from build123d import *

# Parameters (mm, degrees)
SKETCH1_W               = 35
SKETCH1_H               = 54
BOSS_EXTRUDE1_DEPTH     = 12
SKETCH2_W               = 35
SKETCH2_H               = 9
SKETCH2_W_2             = 9
SKETCH2_H_2             = 25
SKETCH2_W_3             = 6
SKETCH2_H_3             = 20
CUT_EXTRUDE1_DEPTH      = 5.5
CUT_EXTRUDE2_DEPTH      = 59.019393309
CUT_EXTRUDE2_DEPTH_BACK = 59.019393309
SKETCH3_W               = 25
SKETCH3_H               = 2
CUT_EXTRUDE3_DEPTH      = 46.803929962
CUT_EXTRUDE3_DEPTH_BACK = 46.803929962
SKETCH4_W               = 8.5
SKETCH4_H               = 2
SKETCH4_W_2             = 26.8
SKETCH4_W_3             = 8.7
FILLET1_R               = 2.5
SKETCH5_W               = 2.5
SKETCH5_H               = 2.389297353
SKETCH5_W_2             = 1.629066377
SKETCH5_H_2             = 1.665267852
SKETCH5_W_3             = 1.411857527
SKETCH5_W_4             = 2.606506203
SKETCH5_H_3             = 1.918678177
BOSS_EXTRUDE2_DEPTH     = 5.5


with BuildPart() as part:
    # Sketch1 → Boss-Extrude1 (new body)
    with BuildSketch(Plane(origin=(0, 0, 0), x_dir=(1, 0, 0), z_dir=(0, 1, 0))):
        Rectangle(SKETCH1_W, SKETCH1_H)
    extrude(amount=BOSS_EXTRUDE1_DEPTH)

    # Sketch2 → Cut-Extrude1 (cut)
    with BuildSketch(Plane(origin=(0, 12, 0), x_dir=(1, 0, 0), z_dir=(0, 1, 0))):
        with Locations((0, -22.5)):
            Rectangle(SKETCH2_W, SKETCH2_H)
        with Locations((-13, 0.5)):
            Rectangle(SKETCH2_W_2, SKETCH2_H_2)
        with Locations((14.5, 3)):
            Rectangle(SKETCH2_W_3, SKETCH2_H_3)
    extrude(amount=-CUT_EXTRUDE1_DEPTH, mode=Mode.SUBTRACT)

    # Sketch3 → Cut-Extrude2 (cut, two sides: drawn at the far end of the back side and taken through both)
    with BuildSketch(Plane(origin=(0, 0, -27), x_dir=(-1, 0, 0), z_dir=(0, 0, -1)).offset(-CUT_EXTRUDE2_DEPTH_BACK)):
        with Locations((0, 2)):
            Rectangle(SKETCH3_W, SKETCH3_H)
    extrude(amount=CUT_EXTRUDE2_DEPTH + CUT_EXTRUDE2_DEPTH_BACK, mode=Mode.SUBTRACT)

    # Sketch4 → Cut-Extrude3 (cut, two sides: drawn at the far end of the back side and taken through both)
    with BuildSketch(Plane.ZY.offset(17.5).offset(-CUT_EXTRUDE3_DEPTH_BACK)):
        with Locations((-22.75, 2)):
            Rectangle(SKETCH4_W, SKETCH4_H)
        with Locations((-0.1, 2)):
            Rectangle(SKETCH4_W_2, SKETCH4_H)
        with Locations((22.65, 2)):
            Rectangle(SKETCH4_W_3, SKETCH4_H)
    extrude(amount=CUT_EXTRUDE3_DEPTH + CUT_EXTRUDE3_DEPTH_BACK, mode=Mode.SUBTRACT)

    # Fillet1
    fillet1_edges = [part.edges().sort_by_distance(p)[0] for p in [
        (12.5, 2, -13.5),
        (12.5, 2, -18.5),
        (17.5, 2, -18.5),
        (17.5, 2, -13.5),
        (12.5, 2, 13.3),
        (12.5, 2, 18.3),
        (17.5, 2, 13.3),
        (17.5, 2, 18.3),
        (-12.5, 2, 13.3),
        (-12.5, 2, 18.3),
        (-12.5, 2, -18.5),
        (-12.5, 2, -13.5),
        (-17.5, 2, 13.3),
        (-17.5, 2, 18.3),
        (-17.5, 2, -18.5),
        (-17.5, 2, -13.5),
    ]]
    fillet(fillet1_edges, radius=FILLET1_R - 0.0001)  # a hair under: the kernel refuses the full size

    # Sketch5 → Boss-Extrude2 (add)
    with BuildSketch(Plane(origin=(0, 0, -27), x_dir=(-1, 0, 0), z_dir=(0, 0, -1))):
        with Locations((-16.25, 5.345369084)):
            Rectangle(SKETCH5_W, SKETCH5_H)
        with Locations((-1.647167115, 5.236764658)):
            Rectangle(SKETCH5_W_2, SKETCH5_H_2)
        with Locations((4.688091019, 5.236764658)):
            Rectangle(SKETCH5_W_3, SKETCH5_H_2)
        with Locations((15.530432797, 5.110059495)):
            Rectangle(SKETCH5_W_4, SKETCH5_H_3)
    extrude(amount=BOSS_EXTRUDE2_DEPTH)


solid = part.part
Model file for the job. Use its own axes, mm. A direction names the side the tool comes from. Give positions to 0.01 mm unless a question says otherwise; leave off trailing zeros. Order: outer loops, then holes, each group sorted by start corner. A loop starts at its lowest first (then second) coordinate and runs counter-clockwise, first axis right, second up. Notation, with made-up numbers: (-16.5, -8) - (5.5, -8) arc R23 cw to (5.5, 4) - close; hole circle Ø10 at (31.25, -26). An arc over 180 degrees is marked (long way). Write item = value, one per line. Start each with the question number.
1. Cut at B-B, the plane x = -10.5. List the corners of the cut face in (y, z), and give its area (3 significant figures).
2. Cut at A-A, the plane z = 10. List the corners of the cut face in (x, y).
3. Cut at C-C, the plane y = 11. List the corners of the cut face in (x, z).
4. Probe line 1 along Y through (x, z) = (2, -8); line 2 along Z through (x, y) = (12.5, 11.75); line 3 along Y through (x, z) = (-15, -11.5). List the from-to ranges inside material, lowest first.
5. Drop flat-ended pins along their axis: P1, Ø0.8, axis at x = -15.5, z = -30, coming from the +Y side; P2, Ø0.8, axis at x = -15.5, z = -29.5, coming from the -Y side; P3, Ø1.6, axis at x = -14.5, y = 8, coming from the +Z side. Give the stop position or say it passes through.
6. Two-plate mould, pull along Z, no slides. Class faces 1 (the flat face through (-5.394, 5, -30)), 2 (the cylindrical face through (-16.787, 1.986, -17.748)), 3 (the cylindrical face through (-16.787, 1.986, 14.052)): pulls with the +Z half, pulls with the -Z half, needs draft (parallel to the pull), parting line crosses it, or undercut.
7. Cut at D-D, the plane z = -4. List the corners of the cut face in (x, y).
8. Which spindle directions (+Z, -Z, +X, -X, +Y, -Y) get a long thin tool onto all of the face, cutting with end or side? Do faces 4 (the cylindrical face through (16.787, 1.986, 14.052)), 5 (the flat face through (-13, 6.5, -1)), 6 (the flat face through (-14.227, 5, -30)). Say none if no direction does.
Taken from the geometry:
q1.outline = (0, -27) - (1, -27) - (1, 27) - (0, 27) - close; (3, -27) - (12, -27) - (12, -13) - (6.5, -13) - (6.5, 12) - (12, 12) - (12, 18) - (6.5, 18) - (6.5, 27) - (3, 27) - close
q1.area = 353 mm²
q2.outline = (-17.5, 0) - (17.5, 0) - (17.5, 1) - (-17.5, 1) - close; (-17.5, 3) - (17.5, 3) - (17.5, 12) - (-8.5, 12) - (-8.5, 6.5) - (-17.5, 6.5) - close
q3.outline = (-17.5, -27) - (17.5, -27) - (17.5, -13) - (11.5, -13) - (11.5, 7) - (17.5, 7) - (17.5, 18) - (-17.5, 18) - (-17.5, 12) - (-8.5, 12) - (-8.5, -13) - (-17.5, -13) - close
q4.line_1 = 0 to 1, 3 to 12
q4.line_2 = -27 to -13, 7 to 18
q4.line_3 = 0 to 1, 3 to 6.5
q5.P1 = 6.07
q5.P2 = 4.15
q5.P3 = 18
q6.face_1 = needs draft
q6.face_2 = pulls with the -Z half
q6.face_3 = undercut
q7.outline = (-17.5, 0) - (17.5, 0) - (17.5, 1) - (-17.5, 1) - close; (-17.5, 3) - (17.5, 3) - (17.5, 6.5) - (11.5, 6.5) - (11.5, 12) - (-8.5, 12) - (-8.5, 6.5) - (-17.5, 6.5) - close
q8.face_4 = +X
q8.face_5 = -X, +Y
q8.face_6 = -Z, +Y, -Y
